from build123d import *

# Parameters (mm, degrees)
SKETCH1_R           = 2
BOSS_EXTRUDE1_DEPTH = 3
SKETCH1_3_R         = 15
SKETCH1_3_R_2       = 2
BOSS_EXTRUDE2_DEPTH = 3


with BuildPart() as part:
    # Sketch1 → Boss-Extrude1 (new body)
    with BuildSketch(Plane(origin=(0, 0, 0), x_dir=(1, 0, 0), z_dir=(0, 1, 0))):
        with BuildLine():
            ThreePointArc((0.5625, -5.973574621), (6, 0), (0.5625, 5.973574621))
            Line((0.5625, 5.973574621), (-94.59375, 14.933936552))
            ThreePointArc((-94.59375, 14.933936552), (-111, 0), (-94.59375, -14.933936552))
            Line((-94.59375, -14.933936552), (0.5625, -5.973574621))
        make_face()
        Circle(SKETCH1_R, mode=Mode.SUBTRACT)
        with Locations((-96, 0)):
            Circle(SKETCH1_R, mode=Mode.SUBTRACT)
        with Locations((-96, 8)):
            Circle(SKETCH1_R, mode=Mode.SUBTRACT)
        with Locations((-96, -8)):
            Circle(SKETCH1_R, mode=Mode.SUBTRACT)
    extrude(amount=BOSS_EXTRUDE1_DEPTH)

    # Sketch1_3 → Boss-Extrude2 (add)
    with BuildSketch(Plane(origin=(0, 0, 0), x_dir=(1, 0, 0), z_dir=(0, 1, 0))):
        with Locations((-96, 0)):
            Circle(SKETCH1_3_R)
        with Locations((-96, 0)):
            Circle(SKETCH1_3_R_2, mode=Mode.SUBTRACT)
        with Locations((-96, 8)):
            Circle(SKETCH1_3_R_2, mode=Mode.SUBTRACT)
        with Locations((-96, -8)):
            Circle(SKETCH1_3_R_2, mode=Mode.SUBTRACT)
    extrude(amount=-BOSS_EXTRUDE2_DEPTH)


solid = part.part
Design review of the part built by this model. Coordinates are the model's own, in mm. Give positions to 0.01 mm unless a question says otherwise; leave off trailing zeros. Loops run counter-clockwise (first coordinate to the right, second up) from the corner with the lowest first, then second, coordinate; pieces in that order, holes last. Notation, with made-up numbers: (-31, 67.25) - (-25, 67.25) arc R27 ccw to (-25, 88.25) - close; hole circle Ø10 at (0, 17.5). An arc over 180 degrees is marked (long way). Use CSV: the item, a comma, the result in double quotes. Start each with the question number.
1. Insertion check: P1, Ø15, axis at x = -50.5, z = -6.5, coming from the -Y side; P2, Ø4.5, axis at x = -96, z = 0, coming from the -Y side; P3, Ø3, axis at y = 2, z = -8.5, coming from the -X side. Each pin has a flat end and moves straight along its axis. Give the tip position at first contact, or say it passes through.
2. Add section C-C (z = 8). State the section outline as (x, y) points.
3. Wall thickness on L1, parallel to X at y = 2.15, z = 0; L2, parallel to Z at x = -96, y = -1.35; L3, parallel to Z at x = -0.5, y = 0.3: over which ranges is each line inside the solid? List them lowest first.
4. Add section D-D (z = -12.5). State the section outline as (x, y) points.
5. Add section B-B (x = -96). State the section outline as (y, z) points.
6. Draft analysis for pull direction X (two halves, no side actions). For faces 1 (the cylindrical face through (0, 1, 2)), 2 (the flat face through (-66, 3, 0)), 3 (the flat face through (-47.682, 1.479, 10.516)), state which applies: released by +X, released by -X, zero draft, split by the parting line, or undercut.
7. Add section A-A (z = 0). State the section outline as (x, y) points.
Results found:
1,P1,"stops at y = 0"
1,P2,"stops at y = -3"
1,P3,"stops at x = -109.27"
2,outline,"(-108.69, -3) - (-98, -3) - (-98, 3) - (-108.69, 3) - close; (-94, -3) - (-83.31, -3) - (-83.31, 0) - (-20.96, 0) - (-20.96, 3) - (-94, 3) - close"
3,L1,"x = -111 to -98, -94 to -2, 2 to 6"
3,L2,"z = -15 to -10, -6 to -2, 2 to 6, 10 to 15"
3,L3,"z = -6.07 to -1.94, 1.94 to 6.07"
4,outline,"(-104.29, -3) - (-87.71, -3) - (-87.71, 0) - (-68.75, 0) - (-68.75, 3) - (-104.29, 3) - close"
5,outline,"(-3, -15) - (3, -15) - (3, -10) - (-3, -10) - close; (-3, -6) - (3, -6) - (3, -2) - (-3, -2) - close; (-3, 2) - (3, 2) - (3, 6) - (-3, 6) - close; (-3, 10) - (3, 10) - (3, 15) - (-3, 15) - close"
6,face 1,"undercut"
6,face 2,"zero draft"
6,face 3,"released by +X"
7,outline,"(-111, -3) - (-98, -3) - (-98, 3) - (-111, 3) - close; (-94, -3) - (-81, -3) - (-81, 0) - (-2, 0) - (-2, 3) - (-94, 3) - close; (2, 0) - (6, 0) - (6, 3) - (2, 3) - close"
